```python
from build123d import *

# Parameters (mm, degrees)
SKETCH1_R           = 60.96
BOSS_EXTRUDE1_DEPTH = 25.4
FILLET1_R           = 2.54
SKETCH2_R           = 4.508
CUT_EXTRUDE1_DEPTH  = 6.35
SKETCH4_R           = 6.35
CUT_EXTRUDE3_DEPTH  = 90.874374546
SKETCH5_R           = 3.175
CUT_EXTRUDE4_DEPTH  = 90.874374546
CIRPATTERN2_COUNT   = 8
SKETCH6_R           = 14.605
CUT_EXTRUDE5_DEPTH  = 22.225
BOSS_EXTRUDE2_START = 6.35
SKETCH7_R           = 14.605
SKETCH7_R_2         = 12.7
BOSS_EXTRUDE2_DEPTH = 6.35
BOSS_EXTRUDE3_START = 8.89
SKETCH8_R           = 17.499965
SKETCH8_R_2         = 14.605
BOSS_EXTRUDE3_DEPTH = 8.89


with BuildPart() as part:
    # Sketch1 → Boss-Extrude1 (new body)
    with BuildSketch(Plane(origin=(0, 0, 0), x_dir=(0, 0, -1), z_dir=(1, 0, 0))):
        Circle(SKETCH1_R)
    extrude(amount=BOSS_EXTRUDE1_DEPTH)

    # Fillet1
    fillet1_edges = [part.edges().sort_by_distance(p)[0] for p in [
        (25.4, 0, 60.96),
    ]]
    fillet(fillet1_edges, radius=FILLET1_R)

    # Sketch2 → Cut-Extrude1 (cut)
    with BuildSketch(Plane(origin=(25.4, 0, 0), x_dir=(0, 0, -1), z_dir=(1, 0, 0))):
        Circle(SKETCH2_R)
    extrude(amount=-CUT_EXTRUDE1_DEPTH, mode=Mode.SUBTRACT)

    # Sketch4 → Cut-Extrude3 (cut, through all)
    with BuildSketch(Plane(origin=(25.4, 0, 0), x_dir=(0, 0, -1), z_dir=(1, 0, 0))):
        Circle(SKETCH4_R)
    extrude(amount=-CUT_EXTRUDE3_DEPTH, mode=Mode.SUBTRACT)

    # Sketch5 → Cut-Extrude4 (cut, through all)
    with BuildSketch(Plane.ZY):
        with Locations((-36.188764222, 35.651274088)):
            Circle(SKETCH5_R)
    cut_extrude4 = extrude(amount=-CUT_EXTRUDE4_DEPTH, mode=Mode.SUBTRACT)

    # CirPattern2: Cut-Extrude4 ×8 about axis, 1 skipped
    cirpattern2_axis = Axis((0, 0, 0), (1, 0, 0))
    add([cut_extrude4.rotate(cirpattern2_axis, i * 360 / CIRPATTERN2_COUNT) for i in range(1, CIRPATTERN2_COUNT) if i not in (7,)], mode=Mode.SUBTRACT)

    # Sketch6 → Cut-Extrude5 (cut)
    with BuildSketch(Plane.ZY):
        Circle(SKETCH6_R)
    extrude(amount=-CUT_EXTRUDE5_DEPTH, mode=Mode.SUBTRACT)

    # Sketch7 → Boss-Extrude2 (add)
    with BuildSketch(Plane.ZY.offset(-22.225).offset(BOSS_EXTRUDE2_START)):
        Circle(SKETCH7_R)
        Circle(SKETCH7_R_2, mode=Mode.SUBTRACT)
    extrude(amount=-BOSS_EXTRUDE2_DEPTH)

    # Sketch8 → Boss-Extrude3 (add)
    with BuildSketch(Plane.ZY.offset(BOSS_EXTRUDE3_START)):
        with Locations(Location((0, 0, 0), (0, 0, 180))):
            Circle(SKETCH8_R)
        Circle(SKETCH8_R_2, mode=Mode.SUBTRACT)
    extrude(amount=-BOSS_EXTRUDE3_DEPTH)


solid = part.part
```
Input: part model. Units: mm. Frame: model coordinates. A direction names the side the tool comes from. Round coordinates to 2 decimals unless told otherwise and drop trailing zeros. Loops run counter-clockwise (first coordinate to the right, second up) from the corner with the lowest first, then second, coordinate; pieces in that order, holes last. Notation, with made-up numbers: M 56.5,19 L 113.5,19 A10 ccw 113.5,34 Z; hole C 40,42 d5. An arc over 180 degrees is marked long. Answer in a Markdown table with one row per item. Add a question column.
1. Ray query, probe 1 along Y at (x, z) = (8, 0) (3 decimals); probe 2 along X at (y, z) = (-22, 37.5); probe 3 along Z at (x, y) = (1, -39). Return the intervals inside material, ascending.
2. Mould query, pull axis Y, two halves, no side actions, for faces 1 (the face through (11.27, -59.51, 13.21)), 2 (the face through (0, -13, -13)), 3 (the face through (19.01, -12.4, -2.75)). Classes: released by +Y, released by -Y, zero draft, split by the parting line, or undercut.
3. Section C-C (y = 0). Output: boundary loops of the cut face in (x, z) (3 decimals).
4. Contact query for flat-ended pins moving along their axis: pin 1 (12 mm diameter, centred on x = 20, y = 29.5, fed in from +Z); pin 2 (6 mm diameter, centred on x = 4, y = 19, fed in from +Z); pin 3 (4 mm diameter, centred on y = -40, z = -22.5, fed in from -X). Output: stop coordinate, or through.
5. Section A-A (z = 0). Give the number of separate pieces and of enclosed holes in the cut face, and give its area (3 significant figures).
6. Set-up query: faces 4 (the face through (15.875, 7, -11)), 5 (the face through (12.522, -36.877, -32.552)). Return all of +Z, -Z, +X, -X, +Y, -Y with unobstructed straight access to the full face (end or side cutting, diameter ignored); none if empty.
Values follow:
| question | item | result |
|---|---|---|
| 1 | probe 1 | -60.96 to -53.951, -47.646 to -14.605, 14.605 to 47.646, 53.951 to 60.96 |
| 1 | probe 2 | 0 to 25.4 |
| 1 | probe 3 | -46.85 to -37.13, -34.18 to 46.85 |
| 2 | face 1 | split by the parting line |
| 2 | face 2 | zero draft |
| 2 | face 3 | undercut |
| 3 | outline | M -8.89,-17.5 L 0,-17.5 L 0,-60.96 L 22.86,-60.96 A2.54 ccw 25.4,-58.42 L 25.4,-6.35 L 22.225,-6.35 L 22.225,-12.7 L 15.875,-12.7 L 15.875,-14.605 L -8.89,-14.605 Z; M -8.89,14.605 L 15.875,14.605 L 15.875,12.7 L 22.225,12.7 L 22.225,6.35 L 25.4,6.35 L 25.4,47.646 L 0,47.646 L 0,17.5 L -8.89,17.5 Z; M 0,53.951 L 25.4,53.951 L 25.4,58.42 A2.54 ccw 22.86,60.96 L 0,60.96 Z |
| 4 | pin 1 | z = 56.25 |
| 4 | pin 2 | z = 58.82 |
| 4 | pin 3 | x = 0 |
| 5 | separate pieces | 4 |
| 5 | enclosed holes | 0 |
| 5 | area | 2,160 mm^2 |
| 6 | face 4 | -X |
| 6 | face 5 | +X, -X |
